Geometry check sheet. Reference: the model listing, model coordinates, mm. Face numbers are marked on the shaded views. Give positions to 0.01 mm unless a question says otherwise; leave off trailing zeros. Loops run counter-clockwise (first coordinate to the right, second up) from the corner with the lowest first, then second, coordinate; pieces in that order, holes last. Notation, with made-up numbers: (87, 66) -> (122, 66) arc R17 cw to (122, 84) -> close; hole circle Ø2 at (-16.5, -7). An arc over 180 degrees is marked (long way). One line per question, with ' | ' between items.
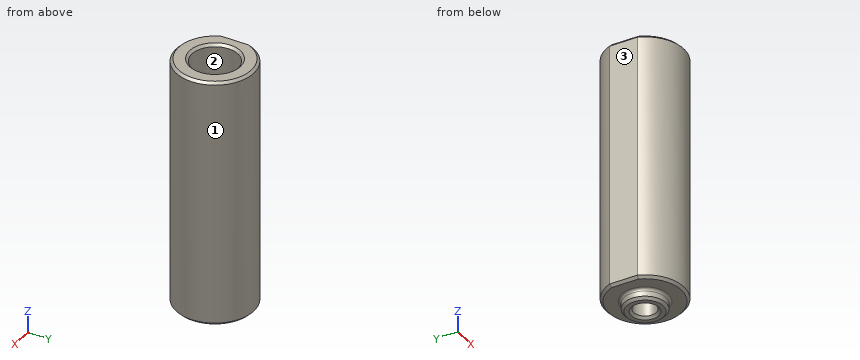
from build123d import *

# Parameters (mm, degrees)
SKETCH1_R                    = 5.95
BOSS_EXTRUDE1_DEPTH          = 38.1
SKETCH2_R                    = 3.175
BOSS_EXTRUDE2_DEPTH          = 1.5875
J_0_277_DIAMETER_HOLE1_D     = 7.0358
J_0_277_DIAMETER_HOLE1_DEPTH = 28.575
J_0_277_DIAMETER_HOLE1_TIP   = 2.113767572
F_8_32_TAPPED_HOLE2_D        = 3.4544
SKETCH9_W                    = 38.1
SKETCH9_H                    = 6
CUT_EXTRUDE3_DEPTH           = 1.396875
CHAMFER1_SIZE                = 0.381
FILLET1_R                    = 0.396875


with BuildPart() as part:
    # Sketch1 → Boss-Extrude1 (new body)
    with BuildSketch(Plane.XY):
        Circle(SKETCH1_R)
    extrude(amount=BOSS_EXTRUDE1_DEPTH)

    # Sketch2 → Boss-Extrude2 (add)
    with BuildSketch(Plane(origin=(0, 0, 0), x_dir=(-1, 0, 0), z_dir=(0, 0, -1))):
        Circle(SKETCH2_R)
    extrude(amount=BOSS_EXTRUDE2_DEPTH)

    # J (0.277) Diameter Hole1
    with Locations(Plane.XY.offset(38.1)):
        with Locations((0, 0)):
            Hole(J_0_277_DIAMETER_HOLE1_D / 2, depth=J_0_277_DIAMETER_HOLE1_DEPTH)
            with Locations((0, 0, -(J_0_277_DIAMETER_HOLE1_DEPTH + J_0_277_DIAMETER_HOLE1_TIP / 2))):  # 118° drill point
                Cone(0, J_0_277_DIAMETER_HOLE1_D / 2, J_0_277_DIAMETER_HOLE1_TIP, mode=Mode.SUBTRACT)

    # #8-32 Tapped Hole2 (through all)
    with Locations(Plane(origin=(0, 0, -1.5875), x_dir=(-1, 0, 0), z_dir=(0, 0, -1))):
        with Locations((0, 0)):
            Hole(F_8_32_TAPPED_HOLE2_D / 2)

    # Sketch9 → Cut-Extrude3 (cut, through all)
    with BuildSketch(Plane.ZY.offset(5.553125)):
        with Locations((19.05, 0)):
            Rectangle(SKETCH9_W, SKETCH9_H)
    extrude(amount=CUT_EXTRUDE3_DEPTH, mode=Mode.SUBTRACT)

    # Chamfer1
    chamfer1_edges = [part.edges().sort_by_distance(p)[0] for p in [
        (3.5179, 0, 38.1),
        (-1.7272, 0, -1.5875),
        (5.95, 0, 0),
        (-5.553125, 0, 0),
        (5.95, 0, 38.1),
        (-5.553125, 0, 38.1),
        (3.175, 0, -1.5875),
    ]]
    chamfer(chamfer1_edges, length=CHAMFER1_SIZE)

    # Fillet1
    fillet1_edges = [part.edges().sort_by_distance(p)[0] for p in [
        (3.175, 0, 0),
    ]]
    fillet(fillet1_edges, radius=FILLET1_R)


solid = part.part
Item 1: Depth check by flat-ended pin: pin 1 Ø1.5 at (x, z) = (-2.5, 6) entering from +Y; pin 2 Ø4 at (x, y) = (0, 0) entering from +Z; pin 3 Ø4 at (x, y) = (0, 0) entering from -Z. Enter the tip coordinate at first touch or a pass-through.
Result:
pin 1: y = 5.69 | pin 2: z = 8.61 | pin 3: z = -1.48
Item 2: Release check for a two-part mould opening along Y. For the marked faces 1, 2 and 3 record: pulls with the +Y half, pulls with the -Y half, needs draft (parallel to the pull), parting line crosses it, or undercut.
Result:
face 1: parting line crosses it | face 2: undercut | face 3: needs draft
Item 3: Sectioned sample at C-C (z = 1). Record the cut outline in (x, y).
Result:
outline: (-5.55, -2.14) arc R5.95 ccw (long way) to (-5.55, 2.14) -> close; hole circle Ø3.45 at (0, 0)
Item 4: Sectioned sample at D-D (z = 21). Record the cut outline in (x, y), plus the area to 3 significant figures.
Result:
outline: (-5.55, -2.14) arc R5.95 ccw (long way) to (-5.55, 2.14) -> close; hole circle Ø7.04 at (0, 0) | area: 71.2 mm2
Item 5: Scan lines: probe 1 along Y at (x, z) = (0, 4.5); probe 2 along Y at (x, z) = (0, 24.5); probe 3 along X at (y, z) = (0, 22.75). Record each from-to range of solid material in increasing order.
Result:
probe 1: -5.95 to -1.73, 1.73 to 5.95 | probe 2: -5.95 to -3.52, 3.52 to 5.95 | probe 3: -5.55 to -3.52, 3.52 to 5.95
